```python
from build123d import *

# Parameters (mm, degrees)
FILLET1_R                        = 1
CBORE_FOR_M2_5_SHCS1_D           = 2.9
CBORE_FOR_M2_5_SHCS1_DEPTH       = 10
CBORE_FOR_M2_5_SHCS1_CBORE_D     = 5.5
CBORE_FOR_M2_5_SHCS1_CBORE_DEPTH = 3
CBORE_FOR_M2_5_SHCS1_TIP         = 0.871247898


with BuildPart() as part:
    # Sketch2 → Revolve1 (revolve)
    with BuildSketch(Plane(origin=(0, -49.046586852, 0), x_dir=(0.998643062566617, 0, 0.052077188744861835), z_dir=(-0.052077188744861835, 0, 0.998643062566617)), mode=Mode.PRIVATE) as revolve1_sk:
        Polygon((-25.6, 4.4), (-22.4, 4.4), (-22.4, 4.584314575), (-24.4, 6.584314575), (-24.4, 8.5), (-48, 8.5), (-48, 0), (-34, 0), (-34, 2), (-27.9, 2), (-27.9, 7), (-25.6, 7), align=None)
    revolve(revolve1_sk.sketch.rotate(Axis((0, -35.16651105, 0), (0, -1, 0)), 267.014846532), axis=Axis((0, -35.16651105, 0), (0, -1, 0)))

    # Fillet1
    fillet1_edges = [part.edges().sort_by_distance(p)[0] for p in [
        (0, -47.046586852, -34),
    ]]
    fillet(fillet1_edges, radius=FILLET1_R)

    # CBORE for M2.5 SHCS1
    with Locations(Plane(origin=(0, -40.546586852, 0), x_dir=(1, 0, 0), z_dir=(0, 1, 0))):
        with Locations((2.135164739, 40.944365565), (40.944365565, -2.135164739), (-40.944365565, 2.135164739), (-2.135164739, -40.944365565)):
            CounterBoreHole(CBORE_FOR_M2_5_SHCS1_D / 2, CBORE_FOR_M2_5_SHCS1_CBORE_D / 2, CBORE_FOR_M2_5_SHCS1_CBORE_DEPTH, depth=CBORE_FOR_M2_5_SHCS1_DEPTH)
            with Locations((0, 0, -(CBORE_FOR_M2_5_SHCS1_DEPTH + CBORE_FOR_M2_5_SHCS1_TIP / 2))):  # 118° drill point
                Cone(0, CBORE_FOR_M2_5_SHCS1_D / 2, CBORE_FOR_M2_5_SHCS1_TIP, mode=Mode.SUBTRACT)


solid = part.part
```
Design review of the part built by this model. Coordinates are the model's own, in mm. A direction names the side the tool comes from. Give positions to 0.01 mm unless a question says otherwise; leave off trailing zeros. Use a Markdown table: item, result. Add a question column.
(1) Machinability: for faces 1 (the face through (-38.404, -42.026, -1.082)), 2 (the face through (-7.49, -47.047, -27.04)), 3 (the face through (-42.327, -46.335, -2.571)), which of the approach directions +Z, -Z, +X, -X, +Y, -Y give a long, thin tool a straight path to every point of the face, cutting with its end or side? Answer none if there is none.
(2) Wall thickness on probe 1 along Z at (x, y) = (-12, -43.5); probe 2 along X at (y, z) = (-43, 13.5); probe 3 along X at (y, z) = (-41.2, 0): over which ranges is each line inside the solid? List them lowest first. Write a range as [from, to].
(3) Mouldability with a two-part tool opening along Z and no side actions: class faces 4 (the face through (3.3, -43.547, -39.8)), 5 (the face through (-22, -40.547, 11)), 6 (the face through (-14.418, -44.856, 45.783)) as +Z half, -Z half, draft (parallel to the pull), parting line (faces both ways), or undercut.
(4) Clearance check with flat-ended pins moving along their axes: P1, Ø4, axis at x = 16.5, y = -41.5, coming from the +Z side; P2, Ø1.6, axis at x = 41.5, z = 1.5, coming from the +Y side; P3, Ø1.5, axis at y = -46.5, z = 17, coming from the +X side; P4, Ø2.5, axis at x = -2.14, z = 40.94, coming from the -Y side. State where each tip first meets the part, or that it passes through.
Report:
| question | item | result |
|---|---|---|
| 1 | face 1 | +Y |
| 1 | face 2 | -Y |
| 1 | face 3 | +Y, -Y |
| 2 | probe 1 | z = [-46.48, -25.19], [-22.61, -20.04], [20.04, 22.61], [25.19, 46.48] |
| 2 | probe 2 | x = [-46.06, -24.42], [-21.75, -19.68], [19.68, 21.75], [24.42, 46.06] |
| 2 | probe 3 | x = [-48, -42.68], [-39.21, -24.4], [24.4, 39.21], [42.68, 48] |
| 3 | face 4 | undercut |
| 3 | face 5 | draft |
| 3 | face 6 | parting line |
| 4 | P1 | stops at z = 45.76 |
| 4 | P2 | stops at y = -43.55 |
| 4 | P3 | stops at x = 45.17 |
| 4 | P4 | passes through |
